Geometry: final body of the model. Coordinates: model frame, mm. Round coordinates to 2 decimals unless told otherwise and drop trailing zeros. Loops run counter-clockwise (first coordinate to the right, second up) from the corner with the lowest first, then second, coordinate; pieces in that order, holes last. Notation, with made-up numbers: (88, -31.75) -> (119, -31.75) arc R8 ccw to (119, -23.75) -> close; hole circle Ø5 at (67, 10). An arc over 180 degrees is marked (long way). Answer in a Markdown table with one row per item.
Autodesk Inventor part; units mm, degrees
ref_plane "YZ Plane" through (0, 0, 0) normal (1, 0, 0) x (0, 1, 0)
ref_plane "XZ Plane" through (0, 0, 0) normal (0, 1, 0) x (-1, 0, 0)
ref_plane "XY Plane" through (0, 0, 0) normal (0, 0, 1) x (1, 0, 0)
sketch "スケッチ1" plane through (0, 0, 0) normal (0, 0, 1) x (1, 0, 0)
  line L0 (0, 0) -> (45, 0)
  line L1 (45, 0) -> (45, 155)
  line L2 (45, 155) -> (0, 155)
  line L3 (0, 155) -> (0, 0)
  dimension "d0" = 155
  dimension "d1" = 45
extrude "押し出し1" add sketch "スケッチ1" along normal blind 5
sketch "スケッチ2" plane through (0, 0, 5) normal (0, 0, 1) x (1, 0, 0)
  line L0 (0, 0) -> (45, 0)
  point P0 (22.6447, 131.5)
  dimension "d4" = 131.5
hole "穴1" at (22.6447, 131.5, 5) direction (0, 0, -1) diameter 24 end through all
sketch "スケッチ3" plane through (0, 0, 0) normal (0, 0, -1) x (-1, 0, 0)
  line L0 (0, 0) -> (-45, 0)
  line L1 (-45, 0) -> (-45, 155)
  line L2 (0, 155) -> (0, 0)
  point P0 (-10, 10)
  point P1 (-35, 10)
  dimension "d12" = 10
  dimension "d13" = 10
  dimension "d14" = 10
  dimension "d15" = 10
hole "穴2" at (10, 10, 0) at (35, 10, 0) direction (0, 0, 1) diameter 5 end through all
properties part number "回転軸取り付け板"
Item 1: Cut plane D-D (x = 30.5). Output: boundary loops of the cut face in (y, z).
Answer:
| item | result |
|---|---|
| outline | (0, 0) -> (122.43, 0) -> (122.43, 5) -> (0, 5) -> close; (140.57, 0) -> (155, 0) -> (155, 5) -> (140.57, 5) -> close |
Item 2: Cut plane B-B (y = 10). Output: boundary loops of the cut face in (x, z), then the cut area to 3 significant figures.
Answer:
| item | result |
|---|---|
| outline | (0, 0) -> (7.5, 0) -> (7.5, 5) -> (0, 5) -> close; (12.5, 0) -> (32.5, 0) -> (32.5, 5) -> (12.5, 5) -> close; (37.5, 0) -> (45, 0) -> (45, 5) -> (37.5, 5) -> close |
| area | 175 mm² |
Item 3: Line query: probe 1 along X at (y, z) = (10, 1.75); probe 2 along Y at (x, z) = (35, 3.6); probe 3 along X at (y, z) = (131.5, 3.9). Output: solid intervals per line, ascending. Write a range as [from, to].
Answer:
| item | result |
|---|---|
| probe 1 | x = [0, 7.5], [12.5, 32.5], [37.5, 45] |
| probe 2 | y = [0, 7.5], [12.5, 155] |
| probe 3 | x = [0, 10.64], [34.64, 45] |
Item 4: Cut plane C-C (z = 3.75). Output: boundary loops of the cut face in (x, y), then the cut area to 3 significant figures.
Answer:
| item | result |
|---|---|
| outline | (0, 0) -> (45, 0) -> (45, 155) -> (0, 155) -> close; hole circle Ø5 at (10, 10); hole circle Ø24 at (22.64, 131.5); hole circle Ø5 at (35, 10) |
| area | 6,480 mm² |
Item 5: Cut plane A-A (y = 131.5). Output: boundary loops of the cut face in (x, z).
Answer:
| item | result |
|---|---|
| outline | (0, 0) -> (10.64, 0) -> (10.64, 5) -> (0, 5) -> close; (34.64, 0) -> (45, 0) -> (45, 5) -> (34.64, 5) -> close |
Item 6: Draft query along Y for faces 1 (the face through (45, 76, 2)), 2 (the face through (22.12, 143.49, 2.46)), 3 (the face through (23, 155, 2)), 4 (the face through (22, 0, 2)). Return one class per face: pulls with the +Y half, pulls with the -Y half, needs draft (parallel to the pull), parting line crosses it, or undercut.
Answer:
| item | result |
|---|---|
| face 1 | needs draft |
| face 2 | undercut |
| face 3 | pulls with the +Y half |
| face 4 | pulls with the -Y half |
Item 7: Pin query (flat end, axial travel): pin 1 Ø1.5 at (x, z) = (36, 3.5) entering from -Y. Return the tip coordinate at first contact, or that it passes through.
Answer:
| item | result |
|---|---|
| pin 1 | stops at y = 0 |
